Build history of the part. All positions in model axes, mm. Face numbers are marked on the shaded views. A direction names the side the tool comes from. Give positions to 0.01 mm unless a question says otherwise; leave off trailing zeros. Write each loop counter-clockwise with the first axis right and the second up, starting at its lowest first coordinate (ties: lowest second). Pieces come first, ordered by that corner, then holes. Notation, with made-up numbers: M 37,1.25 L 60,1.25 A22 cw 60,31.25 Z; hole C 79.5,51 d8. An arc over 180 degrees is marked long. One line per item, written item: value. Start each with the question number.
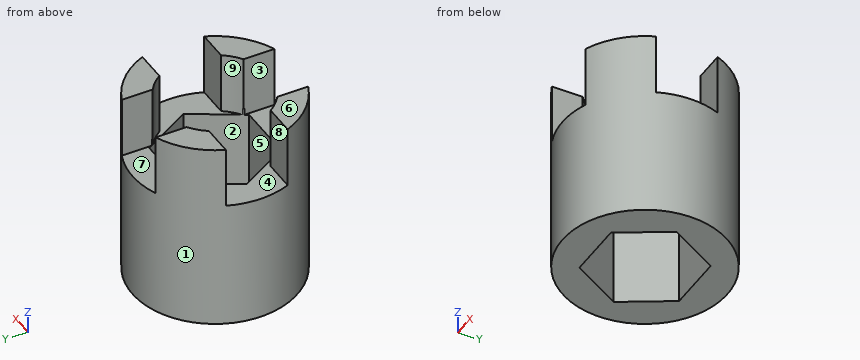
from build123d import *

# Parameters (mm, degrees)
CYLINDER019_R     = 4
CYLINDER019_DEPTH = 4.5
CUBE028_W         = 20
CUBE028_H         = 4.5
CUBE028_DEPTH     = 4.5
CUBE029_W         = 4.5
CUBE029_H         = 20
CUBE029_DEPTH     = 4.5
PRISM022_DEPTH    = 10
CYLINDER018_R     = 6
CYLINDER018_DEPTH = 14


with BuildPart() as cylinder019:
    # cylinder019 → cylinder019 (new body)
    with BuildSketch(Plane(origin=(-66.9, -66.9, -7), x_dir=(1, 0, 0), z_dir=(0, 0, 1))):
        Circle(CYLINDER019_R)
    extrude(amount=CYLINDER019_DEPTH)


with BuildPart() as cube028:
    # cube028 → cube028 (new body)
    with BuildSketch(Plane(origin=(-76.9, -69.15, -7), x_dir=(1, 0, 0), z_dir=(0, 0, 1))):
        with Locations((10, 2.25)):
            Rectangle(CUBE028_W, CUBE028_H)
    extrude(amount=CUBE028_DEPTH)


with BuildPart() as cube029:
    # cube029 → cube029 (new body)
    with BuildSketch(Plane(origin=(-69.15, -76.9, -7), x_dir=(1, 0, 0), z_dir=(0, 0, 1))):
        with Locations((2.25, 10)):
            Rectangle(CUBE029_W, CUBE029_H)
    extrude(amount=CUBE029_DEPTH)


with BuildPart() as group012:
    # prism022 → prism022 (new body)
    with BuildSketch(Plane(origin=(-66.9, -66.9, -16.5), x_dir=(1, 0, 0), z_dir=(0, 0, 1))):
        Polygon((4.2, 0), (2.1, 3.637307), (-2.1, 3.637307), (-4.2, 0), (-2.1, -3.637307), (2.1, -3.637307), align=None)
    extrude(amount=PRISM022_DEPTH)

    # Group012: union cylinder019, cube028, cube029
    add(cylinder019.part)
    add(cube028.part)
    add(cube029.part)


with BuildPart() as nut001:
    # cylinder018 → cylinder018 (new body)
    with BuildSketch(Plane(origin=(-66.9, -66.9, -16.5), x_dir=(1, 0, 0), z_dir=(0, 0, 1))):
        Circle(CYLINDER018_R)
    extrude(amount=CYLINDER018_DEPTH)

    # difference007: cut Group012
    add(group012.part, mode=Mode.SUBTRACT)


solid = nut001.part
1) Band-saw the part on D-D (x = -66.9). List the corners of the cut face in (y, z).
2) Band-saw the part on C-C (y = -68.75). List the corners of the cut face in (x, z), then the cut area to 3 significant figures.
3) Mould opens along Y. For the marked faces 1, 2, 3 and 4 say: released by +Y, released by -Y, zero draft, split by the parting line, or undercut.
4) Tool access for the marked faces 5, 6, 7, 8 and 9: list every direction of +Z, -Z, +X, -X, +Y, -Y with a clear straight run to the whole face (end or side of a thin tool).
5) Band-saw the part on A-A (z = -13.75). List the corners of the cut face in (x, y), then the cut area to 3 significant figures.
6) Probe line 1 along Y through (x, z) = (-67, -14); line 2 along X through (y, z) = (-71, -4.25); line 3 along Y through (x, z) = (-64.25, -12.25). List the from-to ranges inside material, lowest first. Write a range as from..to.
7) Drop flat-ended pins along their axis: P1, Ø1.1, axis at x = -71, z = -5, coming from the -Y side; P2, Ø4, axis at y = -70, z = -13.5, coming from the +X side; P3, Ø2.5, axis at y = -71.5, z = -5, coming from the -X side. Give the stop position or say it passes through.
8) Band-saw the part on B-B (z = -4.25). List the corners of the cut face in (x, y), then the cut area to 3 significant figures.
Model answer:
1. outline: M -72.9,-16.5 L -70.54,-16.5 L -70.54,-7 L -72.9,-7 Z; M -63.26,-16.5 L -60.9,-16.5 L -60.9,-7 L -63.26,-7 Z
2. outline: M -72.61,-16.5 L -70.03,-16.5 L -70.03,-7 L -72.61,-7 Z; M -63.77,-16.5 L -61.19,-16.5 L -61.19,-7 L -63.77,-7 Z
2. area: 48.9 mm²
3. face 1: split by the parting line
3. face 2: undercut
3. face 3: zero draft
3. face 4: undercut
4. face 5: +Z, -Z
4. face 6: +Z, +X, -X, +Y, -Y
4. face 7: +Z, +Y, -Y
4. face 8: +Z, +X, -X
4. face 9: +Z
5. outline: C -66.9,-66.9 d12; hole M -71.1,-66.9 L -69,-70.54 L -64.8,-70.54 L -62.7,-66.9 L -64.8,-63.26 L -69,-63.26 Z
5. area: 67.3 mm²
6. line 1: y = -72.9..-70.54, -63.26..-60.9
6. line 2: x = -71.28..-69.15, -64.65..-62.52
6. line 3: y = -72.28..-69.58, -64.22..-61.52
7. P1: stops at y = -71.74
7. P2: stops at x = -61
7. P3: stops at x = -71.88
8. outline: M -72.46,-69.15 A6 ccw -69.15,-72.46 L -69.15,-70.21 A4 cw -70.21,-69.15 Z; M -72.46,-64.65 L -70.21,-64.65 A4 cw -69.15,-63.59 L -69.15,-61.34 A6 ccw Z; M -64.65,-72.46 A6 ccw -61.34,-69.15 L -63.59,-69.15 A4 cw -64.65,-70.21 Z; M -64.65,-63.59 A4 cw -63.59,-64.65 L -61.34,-64.65 A6 ccw -64.65,-61.34 Z
8. area: 25.4 mm²
